```python
from build123d import *

# Parameters (mm, degrees)
EXTRUDE_2_DEPTH     = 23.3
CUT_EXTRUDE_1_DEPTH = 20.3
SKETCH_5_W          = 18.3
SKETCH_5_H          = 23.3
SKETCH_5_W_2        = 15.3
SKETCH_5_H_2        = 20.3
EXTRUDE_3_DEPTH     = 1.5


with BuildPart() as part:
    # 草圖3 → 填料-伸長2 (new body)
    with BuildSketch(Plane(origin=(0, 0, 0), x_dir=(1, 0, 0), z_dir=(0, 1, 0))):
        with BuildLine():
            Line((-1.5, 0), (16.8, 0))
            Line((16.8, 0), (27.234104494, -7.490738748))
            Line((27.234104494, -7.490738748), (16.8, -13.417750086))
            Line((16.8, -13.417750086), (4.557217445, -8.775105803))
            ThreePointArc((4.557217445, -8.775105803), (0.161354932, -5.331331096), (-1.5, 0))
        make_face()
    extrude(amount=-EXTRUDE_2_DEPTH)

    # 草圖4 → 除料-伸長1 (cut)
    with BuildSketch(Plane(origin=(0, -1.5, 0), x_dir=(1, 0, 0), z_dir=(0, 1, 0))):
        with BuildLine():
            Line((25.798187114, -8.30640037), (15.925221667, -1.21850846))
            ThreePointArc((15.925221667, -1.21850846), (15.465427503, -0.684774598), (15.3, 0))
            Line((15.3, 0), (0, 0))
            ThreePointArc((0, 0), (1.395817627, -4.479214992), (5.089081639, -7.37256508))
            Line((5.089081639, -7.37256508), (18.493554713, -12.455739595))
            Line((18.493554713, -12.455739595), (25.798187114, -8.30640037))
        make_face()
    extrude(amount=-CUT_EXTRUDE_1_DEPTH, mode=Mode.SUBTRACT)

    # 草圖5 → 填料-伸長3 (add)
    with BuildSketch(Plane(origin=(0, 0, 0), x_dir=(-1, 0, 0), z_dir=(0, 0, -1))):
        with Locations((-7.65, -11.65)):
            Rectangle(SKETCH_5_W, SKETCH_5_H)
        with Locations((-7.65, -11.65)):
            Rectangle(SKETCH_5_W_2, SKETCH_5_H_2, mode=Mode.SUBTRACT)
    extrude(amount=EXTRUDE_3_DEPTH)


solid = part.part
```
The listing builds one solid part. Answer for the finished solid, in the listing's coordinates (mm). A direction names the side the tool comes from. Give positions to 0.01 mm unless a question says otherwise; leave off trailing zeros. Write each loop counter-clockwise with the first axis right and the second up, starting at its lowest first coordinate (ties: lowest second). Pieces come first, ordered by that corner, then holes. Notation, with made-up numbers: M 34.25,51.25 L 90.25,51.25 A27 ccw 90.25,82.25 Z; hole C -2,56 d4. An arc over 180 degrees is marked long. Write each question's results on one line, items separated by ' | '.
Q1. For a pull along X with two mould halves and no side action, classify faces 6 (the flat face through (10.764, -11.487, 11.129)), 7 (the flat face through (13, -23.3, 4)), 8 (the flat face through (21.94, -11.49, 3.69)), 9 (the flat face through (20.93, -11.51, 4.81)) as released by +X, released by -X, zero draft, split by the parting line, or undercut.
Output values:
face 6: released by -X | face 7: zero draft | face 8: released by +X | face 9: undercut
Q2. Section B-B, the plane z = 2.25 is taken. Write down the section's boundary in (x, y), then the cut area to 3 significant figures.
Output values:
outline: M -1.23,-23.3 L 19.93,-23.3 L 19.93,0 L -1.23,0 Z; hole M 0.33,-21.8 L 17.36,-21.8 L 17.36,-1.5 L 0.33,-1.5 Z | area: 147 mm2
Q3. Section C-C, the plane x = 22 is taken. Write down the section's boundary in (y, z), then the cut area to 3 significant figures.
Output values:
outline: M -23.3,3.73 L 0,3.73 L 0,10.46 L -1.5,10.46 L -1.5,5.58 L -21.8,5.58 L -21.8,10.46 L -23.3,10.46 Z | area: 57.7 mm2
Q4. Flat-ended cylindrical pins translate along their axes: P1, Ø3, axis at x = 2, z = 7.5, coming from the -Y side; P2, Ø1.2, axis at y = -14, z = -1, coming from the +X side; P3, Ø1.5, axis at x = 14, y = -6, coming from the +Z side; P4, Ø12, axis at x = 24, y = -3, coming from the +Z side. Find the tip coordinate at first contact, or state that the pin passes through.
Output values:
P1: y = -23.3 | P2: x = 16.8 | P3: z = 12.64 | P4: z = 12.74
Q5. A tool of negligible diameter and unlimited length cuts with its end or side. For faces 1 (the flat face through (-0.4, -11.5, -1.5)), 2 (the flat face through (13, -21.8, 6)), 3 (the flat face through (26.727, -11.487, 7.779)), 4 (the flat face through (0, -12, -1)), 5 (the flat face through (16.8, -12, -1)), from which of +Z, -Z, +X, -X, +Y, -Y can it reach the whole face along a straight path? Write none if from no direction.
Output values:
face 1: -Z, +X, -X, +Y, -Y | face 2: none | face 3: +Z, +X, +Y, -Y | face 4: -Z | face 5: -Z, +X, +Y, -Y
Q6. Section A-A, the plane y = -7.5 is taken. Write down the section's boundary in (x, z), then the cut area to 3 significant figures.
Output values:
outline: M -1.5,-1.5 L 0,-1.5 L 0,0 A7.88 cw 5.09,7.37 L 18.49,12.46 L 16.8,13.42 L 4.56,8.78 A9.38 ccw -1.5,0 Z; M 15.3,-1.5 L 16.8,-1.5 L 16.8,0 L 27.23,7.49 L 25.8,8.31 L 15.93,1.22 A1.5 ccw 15.3,0 Z | area: 60.5 mm2
Q7. Consider L1, parallel to Y at x = 24.5, z = 8.5; L2, parallel to X at y = -16.5, z = 6.75; L3, parallel to X at y = -7.5, z = 1.25. Determine where each line is inside the solid, lowest interval first. Write a range as from..to.
Output values:
L1: -23.3..-21.8, -1.5..0 | L2: 1.36..3.81, 23.63..26.2 | L3: -1.42..0.1, 15.97..18.54
Q8. Section D-D, the plane z = 9.5 is taken. Write down the section's boundary in (x, y), then the cut area to 3 significant figures.
Output values:
outline: M 6.47,-23.3 L 23.7,-23.3 L 23.7,-21.8 L 10.7,-21.8 L 10.7,-1.5 L 23.7,-1.5 L 23.7,0 L 6.47,0 Z | area: 138 mm2
